Part model, mm, in its own coordinate system. Coordinates: 2 decimals unless noted, no trailing zeros. Loops run counter-clockwise (first coordinate to the right, second up) from the corner with the lowest first, then second, coordinate; pieces in that order, holes last. Notation, with made-up numbers: M 23,-26.75 L 45,-26.75 A35 cw 45,6.25 Z; hole C 44.5,34 d4. An arc over 180 degrees is marked long. Use a Markdown table: item, result. Add a question column.
1) Wall check: probe 1 along Z at (x, y) = (4, 0.85); probe 2 along Z at (x, y) = (41, 0.8); probe 3 along Z at (x, y) = (59, 2). Give the ranges that are in metal, low to high. Write a range as from..to.
2) Band-saw the part on B-B (z = 53.5). List the corners of the cut face in (x, y), plus the area to 3 significant figures.
3) Pin check, flat tips, straight feed: pin 1 Ø1 at (y, z) = (0.5, -70) entering from -X; pin 2 Ø1.5 at (x, y) = (39, 2) entering from -Z. Stop position of each tip, or through.
4) Band-saw the part on A-A (y = 2.25). List the corners of the cut face in (x, z).
5) Band-saw the part on C-C (x = -11.5). List the corners of the cut face in (y, z), plus the area to 3 significant figures.
Autodesk Inventor part; units mm, degrees
ref_plane "YZ Plane" through (0, 0, 0) normal (1, 0, 0) x (0, 1, 0)
ref_plane "XZ Plane" through (0, 0, 0) normal (0, 1, 0) x (-1, 0, 0)
ref_plane "XY Plane" through (0, 0, 0) normal (0, 0, 1) x (1, 0, 0)
sketch "Sketch1" plane through (0, 0, 0) normal (0, 1, 0) x (-1, 0, 0)
  arc A0 (56.1004, -98.4936) -> (58.4448, -98.4888) centre (57.2693, -96.8707) ccw
  arc A1 (56.1004, -98.4936) -> (-62.636, -98.4936) centre (-3.2678, -180.9204) ccw
  arc A2 (-64.9803, -98.4888) -> (-62.636, -98.4936) centre (-63.8049, -96.8707) ccw
  circle A3 centre (-33.2678, -74.3391) radius 2.5
  circle A4 centre (26.7322, -74.3391) radius 2.5
  circle A5 centre (-43.2678, 76.4616) radius 2.5
  circle A6 centre (36.7322, 76.4616) radius 2.5
  arc A7 (58.4448, -98.4888) -> (-64.9803, -98.4888) centre (-3.2678, -13.5384) ccw
  circle A8 centre (-33.2678, -74.3391) radius 2.5
  circle A9 centre (26.7322, -74.3391) radius 2.5
  circle A10 centre (-33.2678, -74.3391) radius 2.5
  circle A11 centre (26.7322, -74.3391) radius 2.5
  point P0 (0, 0)
  dimension "d25" = 90
  dimension "d26" = 40
  dimension "d27" = 90
  dimension "d28" = 40
extrude "Extrusion5" add sketch "Sketch1" along normal blind 3
properties part number "Middle plate" material "Polycarbonate, Clear"
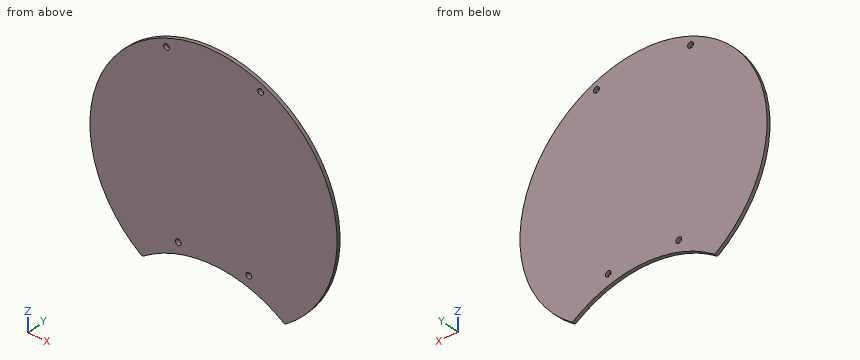
Entries:
| question | item | result |
|---|---|---|
| 1 | probe 1 | -79.34..91.46 |
| 1 | probe 2 | -86.61..75.41, 77.51..84.45 |
| 1 | probe 3 | -95.99..75.45 |
| 2 | outline | M -77.55,0 L 84.08,0 L 84.08,3 L -77.55,3 Z |
| 2 | area | 485 mm2 |
| 3 | pin 1 | x = -85.58 |
| 3 | pin 2 | z = -86.12 |
| 4 | outline | M -58.44,-98.49 A2 ccw -56.1,-98.49 A101.58 cw 62.64,-98.49 A2 ccw 64.98,-98.49 A105 ccw long Z; hole C -36.73,76.46 d5; hole C -26.73,-74.34 d5; hole C 33.27,-74.34 d5; hole C 43.27,76.46 d5 |
| 5 | outline | M 0,-80.42 L 3,-80.42 L 3,90.42 L 0,90.42 Z |
| 5 | area | 513 mm2 |
